Here's how the part is built. I have some questions about the finished solid (model axes, mm). Face numbers are marked on the shaded views. A direction names the side the tool comes from. Coordinates: 2 decimals unless noted, no trailing zeros. Write each loop counter-clockwise with the first axis right and the second up, starting at its lowest first coordinate (ties: lowest second). Pieces come first, ordered by that corner, then holes.
Item 1: If we section it at A-A (x = 33.5): Please give me the cut outline in (y, z).
Item 2: If we section it at C-C (z = 24.5): Please give me the cut outline in (x, y).
Item 3: If we section it at B-B (y = 17): Please give me the cut outline in (x, z).
Item 4: We'd pull the mould along X, two halves only. Please class the marked faces 1 and 2: +X half, -X half, draft (parallel to the pull), parting line (faces both ways), or undercut.
Item 5: If we section it at D-D (x = -30): Please give me the cut outline in (y, z).
Item 6: For the marked faces 3 and 4, which set-ups out of +Z, -Z, +X, -X, +Y, -Y let a thin tool reach every point of the face, with its end or its side?
Item 7: If I drill on line 1 (Y direction, x = 3, z = 27); line 2 (Z direction, x = -31, y = 6.5); line 3 (X direction, y = 16, z = -7), over which ranges is the centre line in solid material (lowest first)?
Item 8: I'm going to push flat-ended pins straight in: pin 1 Ø7.5 at (x, y) = (6.5, 24) entering from -Z; pin 2 Ø1.2 at (y, z) = (6.5, -26.5) entering from +X; pin 3 Ø8 at (x, z) = (4.5, -28.5) entering from -Y. Where does each tip first touch, or does it pass through?
from build123d import *

# Parameters (mm, degrees)
BOSS_EXTRU_1_DEPTH      = 3
ESQUISSE2_R             = 1.5
ENL_V_MAT_EXTRU_1_DEPTH = 3
ESQUISSE3_W             = 75
ESQUISSE3_H             = 85
BOSS_EXTRU_2_DEPTH      = 8
ESQUISSE5_W             = 75
ESQUISSE5_H             = 58
BOSS_EXTRU_4_DEPTH      = 20
ESQUISSE6_R             = 3.783823372
ENL_V_MAT_EXTRU_2_DEPTH = 1
ESQUISSE8_W             = 65
ESQUISSE8_H             = 8
ESQUISSE8_H_2           = 5
ENL_V_MAT_EXTRU_3_DEPTH = 86
ESQUISSE9_W             = 58
ESQUISSE9_H             = 8
ESQUISSE9_H_2           = 5
ENL_V_MAT_EXTRU_4_DEPTH = 1
ESQUISSE10_W            = 58
ESQUISSE10_H            = 5.00265017
ESQUISSE10_H_2          = 8
ENL_V_MAT_EXTRU_5_DEPTH = 1
ESQUISSE11_W            = 4
ESQUISSE11_H            = 5
ESQUISSE11_H_2          = 8
ENL_V_MAT_EXTRU_6_DEPTH = 1
ESQUISSE12_W            = 4
ESQUISSE12_H            = 5
ESQUISSE12_H_2          = 8
ESQUISSE12_H_3          = 5.00265017
ENL_V_MAT_EXTRU_7_DEPTH = 1
ESQUISSE13_W            = 33.774018013
ESQUISSE13_H            = 51.072823149
ENL_V_MAT_EXTRU_8_DEPTH = 8
ESQUISSE14_W            = 20.555972115
ESQUISSE14_H            = 1.5
ESQUISSE14_W_2          = 21.85857566
ESQUISSE14_W_3          = 24.585452225
ENL_V_MAT_EXTRU_9_DEPTH = 8
ESQUISSE15_W            = 8.195150742
ESQUISSE15_H            = 9.302603545
BOSS_EXTRU_5_DEPTH      = 3


with BuildPart() as part:
    # Esquisse1 → Boss.-Extru.1 (new body)
    with BuildSketch(Plane(origin=(0, 0, 0), x_dir=(1, 0, 0), z_dir=(0, 1, 0))):
        Polygon((-53.560263118, 14.694067924), (-43.639645315, 18.536411574), (41.360354685, 18.536411574), (51.439736882, 12.378755225), (51.439736882, -38.621244775), (41.519119079, -42.463588426), (-43.480880921, -42.463588426), (-53.560263118, -36.305932076), align=None)
    extrude(amount=BOSS_EXTRU_1_DEPTH)

    # Esquisse2 → Enlèv. mat.-Extru.1 (cut)
    with BuildSketch(Plane(origin=(0, 3, 0), x_dir=(1, 0, 0), z_dir=(0, 1, 0))):
        with Locations((39.381313418, 10.536411574)):
            Circle(ESQUISSE2_R)
        with Locations((-41.618686582, 10.536411574)):
            Circle(ESQUISSE2_R)
        with Locations((-23.999021885, -35.463588426)):
            Circle(ESQUISSE2_R)
        with Locations((22.000978115, -35.463588426)):
            Circle(ESQUISSE2_R)
    extrude(amount=-ENL_V_MAT_EXTRU_1_DEPTH, mode=Mode.SUBTRACT)

    # Esquisse3 → Boss.-Extru.2 (add)
    with BuildSketch(Plane(origin=(0, 3, 0), x_dir=(1, 0, 0), z_dir=(0, 1, 0))):
        with Locations((-1.060263118, 10.036411574)):
            Rectangle(ESQUISSE3_W, ESQUISSE3_H)
    extrude(amount=BOSS_EXTRU_2_DEPTH)

    # Esquisse5 → Boss.-Extru.4 (add)
    with BuildSketch(Plane(origin=(0, 11, 0), x_dir=(1, 0, 0), z_dir=(0, 1, 0))):
        with Locations((-1.060263118, -3.463588426)):
            Rectangle(ESQUISSE5_W, ESQUISSE5_H)
    extrude(amount=BOSS_EXTRU_4_DEPTH)

    # Esquisse6 → Enlèv. mat.-Extru.2 (cut)
    with BuildSketch(Plane.XZ):
        with Locations((-1.060263118, 13.121244775)):
            Circle(ESQUISSE6_R)
    extrude(amount=-ENL_V_MAT_EXTRU_2_DEPTH, mode=Mode.SUBTRACT)

    # Esquisse8 → Enlèv. mat.-Extru.3 (cut)
    with BuildSketch(Plane(origin=(0, 0, -25.536411574), x_dir=(-1, 0, 0), z_dir=(0, 0, -1))):
        with Locations((1.060263118, 15)):
            Rectangle(ESQUISSE8_W, ESQUISSE8_H)
        with Locations((1.060263118, 28.5)):
            Rectangle(ESQUISSE8_W, ESQUISSE8_H_2)
    extrude(amount=-ENL_V_MAT_EXTRU_3_DEPTH, mode=Mode.SUBTRACT)

    # Esquisse9 → Enlèv. mat.-Extru.4 (cut)
    with BuildSketch(Plane.ZY.offset(38.560263118)):
        with Locations((3.463588426, 15)):
            Rectangle(ESQUISSE9_W, ESQUISSE9_H)
        with Locations((3.463588426, 28.5)):
            Rectangle(ESQUISSE9_W, ESQUISSE9_H_2)
    extrude(amount=-ENL_V_MAT_EXTRU_4_DEPTH, mode=Mode.SUBTRACT)

    # Esquisse10 → Enlèv. mat.-Extru.5 (cut)
    with BuildSketch(Plane(origin=(36.439736882, 0, 0), x_dir=(0, 0, -1), z_dir=(1, 0, 0))):
        with Locations((-3.463588426, 28.498674915)):
            Rectangle(ESQUISSE10_W, ESQUISSE10_H)
        with Locations((-3.463588426, 15)):
            Rectangle(ESQUISSE10_W, ESQUISSE10_H_2)
    extrude(amount=-ENL_V_MAT_EXTRU_5_DEPTH, mode=Mode.SUBTRACT)

    # Esquisse11 → Enlèv. mat.-Extru.6 (cut)
    with BuildSketch(Plane(origin=(0, 0, -25.536411574), x_dir=(-1, 0, 0), z_dir=(0, 0, -1))):
        with Locations((-33.439736882, 28.5)):
            Rectangle(ESQUISSE11_W, ESQUISSE11_H)
        with Locations((-33.439736882, 15)):
            Rectangle(ESQUISSE11_W, ESQUISSE11_H_2)
        with Locations((35.560263118, 15)):
            Rectangle(ESQUISSE11_W, ESQUISSE11_H_2)
        with Locations((35.560263118, 28.5)):
            Rectangle(ESQUISSE11_W, ESQUISSE11_H)
    extrude(amount=-ENL_V_MAT_EXTRU_6_DEPTH, mode=Mode.SUBTRACT)

    # Esquisse12 → Enlèv. mat.-Extru.7 (cut)
    with BuildSketch(Plane.XY.offset(32.463588426)):
        with Locations((-35.560263118, 28.5)):
            Rectangle(ESQUISSE12_W, ESQUISSE12_H)
        with Locations((-35.560263118, 15)):
            Rectangle(ESQUISSE12_W, ESQUISSE12_H_2)
        with Locations((33.439736882, 28.498674915)):
            Rectangle(ESQUISSE12_W, ESQUISSE12_H_3)
        with Locations((33.439736882, 15)):
            Rectangle(ESQUISSE12_W, ESQUISSE12_H_2)
    extrude(amount=-ENL_V_MAT_EXTRU_7_DEPTH, mode=Mode.SUBTRACT)

    # Esquisse13 → Enlèv. mat.-Extru.8 (cut)
    with BuildSketch(Plane(origin=(0, 26, 0), x_dir=(1, 0, 0), z_dir=(0, 1, 0))):
        with Locations((-1.560263118, 25.536411575)):
            Rectangle(ESQUISSE13_W, ESQUISSE13_H)
    extrude(amount=-ENL_V_MAT_EXTRU_8_DEPTH, mode=Mode.SUBTRACT)

    # Esquisse14 → Enlèv. mat.-Extru.9 (cut)
    with BuildSketch(Plane(origin=(0, 11, 0), x_dir=(1, 0, 0), z_dir=(0, 1, 0))):
        with Locations((-28.282277061, 26.286411574)):
            Rectangle(ESQUISSE14_W, ESQUISSE14_H)
        with Locations((25.510449052, 26.286411574)):
            Rectangle(ESQUISSE14_W_2, ESQUISSE14_H)
        with Locations((-1.711564891, 26.286411574)):
            Rectangle(ESQUISSE14_W_3, ESQUISSE14_H)
    extrude(amount=-ENL_V_MAT_EXTRU_9_DEPTH, mode=Mode.SUBTRACT)

    # Esquisse15 → Boss.-Extru.5 (add)
    with BuildSketch(Plane(origin=(0, 11, 0), x_dir=(1, 0, 0), z_dir=(0, 1, 0))):
        with Locations((24.189660789, 52.656882102)):
            Rectangle(ESQUISSE15_W, ESQUISSE15_H)
    extrude(amount=BOSS_EXTRU_5_DEPTH)


solid = part.part
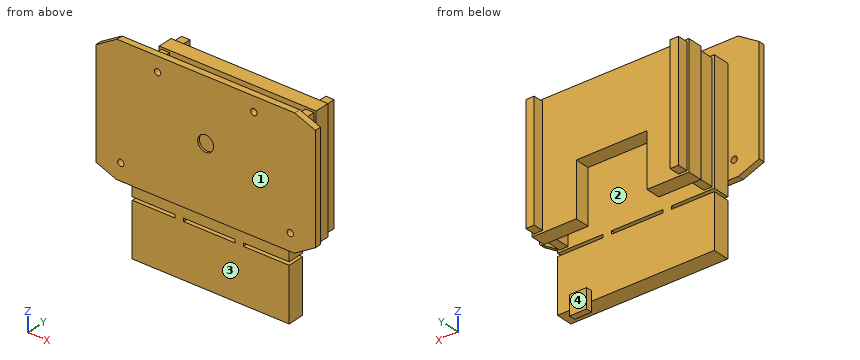
Answer list:
1. outline: (0, -18.54) - (3, -18.54) - (3, -25.54) - (11, -25.54) - (11, -24.54) - (19, -24.54) - (19, -25.54) - (26, -25.54) - (26, -24.54) - (31, -24.54) - (31, 31.46) - (26, 31.46) - (26, 32.46) - (19, 32.46) - (19, 31.46) - (11, 31.46) - (11, 32.46) - (3, 32.46) - (3, 42.46) - (0, 42.46) - close; (3, -52.54) - (11, -52.54) - (11, -27.04) - (3, -27.04) - close
2. outline: (-53.56, 0) - (51.44, 0) - (51.44, 3) - (36.44, 3) - (36.44, 11) - (35.44, 11) - (35.44, 19) - (36.44, 19) - (36.44, 26) - (35.44, 26) - (35.44, 31) - (31.44, 31) - (31.44, 26) - (-33.56, 26) - (-33.56, 31) - (-37.56, 31) - (-37.56, 26) - (-38.56, 26) - (-38.56, 19) - (-37.56, 19) - (-37.56, 11) - (-38.56, 11) - (-38.56, 3) - (-53.56, 3) - close; hole (-33.56, 11) - (31.44, 11) - (31.44, 19) - (-33.56, 19) - close
3. outline: (-37.56, -24.54) - (-33.56, -24.54) - (-33.56, 31.46) - (-37.56, 31.46) - close; (31.44, -24.54) - (35.44, -24.54) - (35.44, 31.46) - (31.44, 31.46) - close
4. face 1: draft
4. face 2: undercut
5. outline: (0, -18.54) - (3, -18.54) - (3, -25.54) - (11, -25.54) - (11, 32.46) - (3, 32.46) - (3, 42.46) - (0, 42.46) - close; (3, -52.54) - (11, -52.54) - (11, -27.04) - (3, -27.04) - close; (19, -25.54) - (26, -25.54) - (26, 32.46) - (19, 32.46) - close
6. face 3: -Z, +X, -X, -Y
6. face 4: +Z, -Z, +X, -X, +Y
7. line 1: y = 0 to 11, 19 to 26
7. line 2: z = -52.54 to -27.04, -25.54 to 32.46
7. line 3: x = -37.56 to -33.56, 31.44 to 35.44
8. pin 1: stops at z = 0
8. pin 2: stops at x = 36.44
8. pin 3: stops at y = 3
